Input: part model. Units: mm. Frame: model coordinates. A direction names the side the tool comes from. Give positions to 0.01 mm unless a question says otherwise; leave off trailing zeros. Write each loop counter-clockwise with the first axis right and the second up, starting at its lowest first coordinate (ties: lowest second). Pieces come first, ordered by that corner, then holes. Notation, with made-up numbers: (30, -21) -> (53, -21) arc R14 ccw to (53, -6) -> close; hole circle Ø9 at (48, -11). An arc over 180 degrees is marked (long way). Answer as a JSON object with one key per item and string values. Group by question number.
from build123d import *

# Parameters (mm, degrees)
SKETCH009_W         = 30.5
SKETCH009_H         = 187.185136
EXTRUDE005_DEPTH    = 40
REVOLUTION001_ANGLE = 180


with BuildPart() as extrude005:
    # Sketch009 → Extrude005 (new body)
    with BuildSketch(Plane(origin=(22, 23, 10), x_dir=(0, 0, -1), z_dir=(0, 1, 0))):
        with Locations((-15.25, 27)):
            Rectangle(SKETCH009_W, SKETCH009_H)
    extrude(amount=EXTRUDE005_DEPTH)


with BuildPart() as cut004:
    # Sketch002 → Revolution001 (revolve)
    with BuildSketch(Plane.XZ):
        Polygon((32.5, 50), (15, 32.5), (15, 17.5), (32.5, 0), (47.5, 0), (47.5, 50), align=None)
    revolve(axis=Axis((0, 0, 0), (0, 0, 1)), revolution_arc=REVOLUTION001_ANGLE)

    # Cut004: cut Extrude005
    add(extrude005.part, mode=Mode.SUBTRACT)


solid = cut004.part
1. Section D-D (z = 11). Return the cut outline in (x, y).
2. Section A-A (y = 40.5). Return the cut outline in (x, z), plus the area to 3 significant figures.
3. Line query: line 1 (Z direction, x = -5, y = 33); line 2 (Y direction, x = -28, z = 13); line 3 (X direction, y = 21, z = 43). Output: solid intervals per line, ascending.
4. Section C-C (x = -37). Return the cut outline in (y, z), plus the area to 3 significant figures.
5. Reachability of faces 1 (the face through (1, 32, 10)), 2 (the face through (-1, 35, 50)) from +Z, -Z, +X, -X, +Y, -Y: full face, straight path, thin tool, end or side. Return the list, or none.
6. Mould query, pull axis Z, two halves, no side actions, for faces 3 (the face through (-1, 23, 25)), 4 (the face through (1, 35, 0)), 5 (the face through (35, 0, 25)). Classes: pulls with the +Z half, pulls with the -Z half, needs draft (parallel to the pull), parting line crosses it, or undercut.
7. Section B-B (z = 33.5). Return the cut outline in (x, y).
8. Contact query for flat-ended pins moving along their axis: pin 1 Ø3 at (x, z) = (-36.5, 18.5) entering from +Y; pin 2 Ø8 at (x, y) = (-7.5, 10) entering from +Z; pin 3 Ø12 at (y, z) = (40.5, 6.5) entering from -X; pin 4 Ø1.5 at (x, y) = (-11.5, 6.5) entering from +Z (1 decimal). Output: stop coordinate, or through.
Working result:
{
 "1": {"outline": "(-47.5, 0) -> (-21.5, 0) arc R21.5 cw to (21.5, 0) -> (47.5, 0) arc R47.5 ccw to (41.56, 23) -> (-41.56, 23) arc R47.5 ccw to start"},
 "2": {"outline": "(-24.82, 0) -> (24.82, 0) -> (24.82, 10) -> (-24.82, 10) -> close; (-24.82, 40.5) -> (24.82, 40.5) -> (24.82, 50) -> (-24.82, 50) -> close", "area": "968 mm^2"},
 "3": {"line 1": "z = 0 to 10, 40.5 to 50", "line 2": "y = 0 to 23", "line 3": "x = -42.61 to -14.47, 14.47 to 42.61"},
 "4": {"outline": "(0, 0) -> (29.79, 0) -> (29.79, 10) -> (23, 10) -> (23, 40.5) -> (29.79, 40.5) -> (29.79, 50) -> (0, 50) -> close", "area": "1,280 mm^2"},
 "5": {"face 1": "+X, -X, +Y", "face 2": "+Z, +X, -X, +Y, -Y"},
 "6": {"face 3": "undercut", "face 4": "pulls with the -Z half", "face 5": "needs draft"},
 "7": {"outline": "(-47.5, 0) -> (-16, 0) arc R16 cw to (16, 0) -> (47.5, 0) arc R47.5 ccw to (41.56, 23) -> (-41.56, 23) arc R47.5 ccw to start"},
 "8": {"pin 1": "stops at y = 23", "pin 2": "stops at z = 34", "pin 3": "stops at x = -32.65", "pin 4": "passes through"}
}
